from build123d import *

# Parameters (mm, degrees)
ESTRUSIONE_ESTRUSIONE1_DEPTH = 15
SCHIZZO6_R                   = 3
TAGLIO_ESTRUSIONE1_DEPTH     = 10
FORO_FILETTATO_M3_1_D        = 2.5


with BuildPart() as part:
    # Schizzo1 → Estrusione-Estrusione1 (new body)
    with BuildSketch(Plane(origin=(0, 0, 0), x_dir=(1, 0, 0), z_dir=(0, 1, 0))):
        Polygon((8, -7), (20, -7), (20, 0), (0, 0), (0, -20), (8, -20), align=None)
    extrude(amount=ESTRUSIONE_ESTRUSIONE1_DEPTH)

    # Schizzo6 → Taglio-Estrusione1 (cut)
    with BuildSketch(Plane(origin=(0, 0, 0), x_dir=(-1, 0, 0), z_dir=(0, 0, -1))):
        with Locations((-16, 7.5)):
            Circle(SCHIZZO6_R)
    extrude(amount=-TAGLIO_ESTRUSIONE1_DEPTH, mode=Mode.SUBTRACT)

    # Foro filettato M3-1 (through all)
    with Locations(Plane(origin=(4, 15, 16.5), x_dir=(0, 0, 1), z_dir=(0, 1, 0))):
        with Locations((0, 0)):
            Hole(FORO_FILETTATO_M3_1_D / 2)


solid = part.part
CAD build for the part. Positions are in the model's coordinates, mm. A direction names the side the tool comes from. Round coordinates to 2 decimals unless told otherwise and drop trailing zeros. Write each loop counter-clockwise with the first axis right and the second up, starting at its lowest first coordinate (ties: lowest second). Pieces come first, ordered by that corner, then holes.
(1) Mould opens along X. For faces 1 (the face through (7.6, 15, 7.6)), 2 (the face through (0, 7, 10)), 3 (the face through (19, 7.6, 3.5)) say: pulls with the +X half, pulls with the -X half, needs draft (parallel to the pull), parting line crosses it, or undercut.
(2) Slice it at C-C, the plane z = 5. Write the cut outline in (x, y), and give its area (3 significant figures).
(3) Probe line 1 along Y through (x, z) = (16, 2.25); line 2 along X through (y, z) = (6.75, 16.5); line 3 along Z through (x, y) = (13, 4). List the from-to ranges inside material, lowest first.
(4) Drop flat-ended pins along their axis: P1, Ø1.5, axis at x = 4, z = 16.5, coming from the +Y side; P2, Ø4, axis at y = 7, z = 12.5, coming from the +X side. Give the stop position or say it passes through.
(5) 3-axis set-ups, long thin cutter, end or side, ignore diameter. For faces 4 (the face through (20, 7, 4)), 5 (the face through (12.6, 7.4, 7)): which of +Z, -Z, +X, -X, +Y, -Y reach the whole face in a straight line?
(6) Slice it at A-A, the plane y = 7.5. Write the cut outline in (x, z), and give its area (3 significant figures).
(7) Slice it at D-D, the plane y = 1.5. Write the cut outline in (x, z), and give its area (3 significant figures).
(8) Slice it at B-B, the plane x = 4. Write the cut outline in (y, z), and give its area (4 significant figures).
From the geometry:
1. face 1: needs draft
1. face 2: pulls with the -X half
1. face 3: undercut
2. outline: (0, 0) - (20, 0) - (20, 15) - (0, 15) - close; hole circle Ø6 at (16, 7.5)
2. area: 272 mm2
3. line 1: y = 0 to 4.5, 10.5 to 15
3. line 2: x = 0 to 2.75, 5.25 to 8
3. line 3: z = 0 to 7
4. P1: passes through
4. P2: stops at x = 8
5. face 4: +Z, -Z, +X, +Y, -Y
5. face 5: +Z, +X, +Y, -Y
6. outline: (0, 0) - (13, 0) - (13, 7) - (8, 7) - (8, 20) - (0, 20) - close; (19, 0) - (20, 0) - (20, 7) - (19, 7) - close; hole circle Ø2.5 at (4, 16.5)
6. area: 197 mm2
7. outline: (0, 0) - (20, 0) - (20, 7) - (8, 7) - (8, 20) - (0, 20) - close; hole circle Ø2.5 at (4, 16.5)
7. area: 239 mm2
8. outline: (0, 0) - (15, 0) - (15, 15.25) - (0, 15.25) - close; (0, 17.75) - (15, 17.75) - (15, 20) - (0, 20) - close
8. area: 262.5 mm2
